```python
from build123d import *

# Parameters (mm, degrees)
BOSS_EXTRUDE1_DEPTH    = 57.15
F_10_32_TAPPED_HOLE1_D = 4.0386


with BuildPart() as part:
    # Sketch1 → Boss-Extrude1 (new body)
    with BuildSketch(Plane(origin=(0, 0, 0), x_dir=(1, 0, 0), z_dir=(0, 1, 0))):
        with BuildLine():
            Line((-4.445, 9.525), (4.445, 9.525))
            ThreePointArc((4.445, 9.525), (8.037102448, 8.037102448), (9.525, 4.445))
            Line((9.525, 4.445), (9.525, -4.445))
            ThreePointArc((9.525, -4.445), (8.037102448, -8.037102448), (4.445, -9.525))
            Line((4.445, -9.525), (-4.445, -9.525))
            ThreePointArc((-4.445, -9.525), (-8.037102448, -8.037102448), (-9.525, -4.445))
            Line((-9.525, -4.445), (-9.525, 4.445))
            ThreePointArc((-9.525, 4.445), (-8.037102448, 8.037102448), (-4.445, 9.525))
        make_face()
    extrude(amount=BOSS_EXTRUDE1_DEPTH)

    # #10-32 Tapped Hole1 (through all)
    with Locations(Plane.XY.offset(9.525)):
        with Locations((0, 44.45), (0, 12.7)):
            Hole(F_10_32_TAPPED_HOLE1_D / 2)


solid = part.part
```
Could you check a few things on this model? Use its own coordinates, in mm. Coordinates: 2 decimals unless noted, no trailing zeros. Write each loop counter-clockwise with the first axis right and the second up, starting at its lowest first coordinate (ties: lowest second). Pieces come first, ordered by that corner, then holes. Notation, with made-up numbers: (21, 42.5) - (42, 42.5) arc R27 ccw to (42, 61.5) - close; hole circle Ø10 at (41.25, 68.25). An arc over 180 degrees is marked (long way). Use a Markdown table: item, result.
Q1. Imagine slicing it at A-A (y = 44.45). List the corners of the cut face in (x, z) for me (3 decimals), and give its area (3 significant figures).
Geometry check:
| item | result |
|---|---|
| outline | (-9.525, -4.445) arc R5.08 ccw to (-4.445, -9.525) - (-2.019, -9.525) - (-2.019, 9.525) - (-4.445, 9.525) arc R5.08 ccw to (-9.525, 4.445) - close; (2.019, -9.525) - (4.445, -9.525) arc R5.08 ccw to (9.525, -4.445) - (9.525, 4.445) arc R5.08 ccw to (4.445, 9.525) - (2.019, 9.525) - close |
| area | 264 mm2 |
Q2. Please list where these lines run through material, in increasing order: L1, parallel to Y at x = 0, z = -0.25; L2, parallel to Y at x = 1, z = 3.5; L3, parallel to Z at x = -4.75, y = 51.
Geometry check:
| item | result |
|---|---|
| L1 | y = 0 to 10.68, 14.72 to 42.43, 46.47 to 57.15 |
| L2 | y = 0 to 10.95, 14.45 to 42.7, 46.2 to 57.15 |
| L3 | z = -9.52 to 9.52 |
Q3. Imagine slicing it at C-C (x = 0). List the corners of the cut face in (y, z) for me (3 decimals), and give its area (3 significant figures).
Geometry check:
| item | result |
|---|---|
| outline | (0, -9.525) - (10.681, -9.525) - (10.681, 9.525) - (0, 9.525) - close; (14.719, -9.525) - (42.431, -9.525) - (42.431, 9.525) - (14.719, 9.525) - close; (46.469, -9.525) - (57.15, -9.525) - (57.15, 9.525) - (46.469, 9.525) - close |
| area | 935 mm2 |
Q4. I'm going to push flat-ended pins straight in: pin 1 Ø3 at (x, y) = (0, 44.45) entering from +Z; pin 2 Ø1.5 at (x, y) = (7, 11.5) entering from -Z. Where does each tip first touch, or does it pass through?
Geometry check:
| item | result |
|---|---|
| pin 1 | passes through |
| pin 2 | stops at z = -9.19 |
Q5. Imagine slicing it at B-B (z = 2). List the corners of the cut face in (x, y) for me (3 decimals), and give its area (3 significant figures).
Geometry check:
| item | result |
|---|---|
| outline | (-9.525, 0) - (9.525, 0) - (9.525, 57.15) - (-9.525, 57.15) - close; hole circle Ø4.039 at (0, 12.7); hole circle Ø4.039 at (0, 44.45) |
| area | 1,060 mm2 |
Q6. Imagine slicing it at D-D (y = 52). List the corners of the cut face in (x, z) for me (3 decimals).
Geometry check:
| item | result |
|---|---|
| outline | (-9.525, -4.445) arc R5.08 ccw to (-4.445, -9.525) - (4.445, -9.525) arc R5.08 ccw to (9.525, -4.445) - (9.525, 4.445) arc R5.08 ccw to (4.445, 9.525) - (-4.445, 9.525) arc R5.08 ccw to (-9.525, 4.445) - close |
Q7. Thinking about a two-plate mould opening in Y: for faces 1 (the flat face through (9.525, 28, 0)), 2 (the flat face through (0, 57.15, 0)), 3 (the cylindrical face through (0.44, 10.73, -0.13)), 4 (the flat face through (0, 0, 0)), which applies, +Y half, -Y half, draft (parallel to the pull), parting line (faces both ways), or undercut?
Geometry check:
| item | result |
|---|---|
| face 1 | draft |
| face 2 | +Y half |
| face 3 | undercut |
| face 4 | -Y half |
